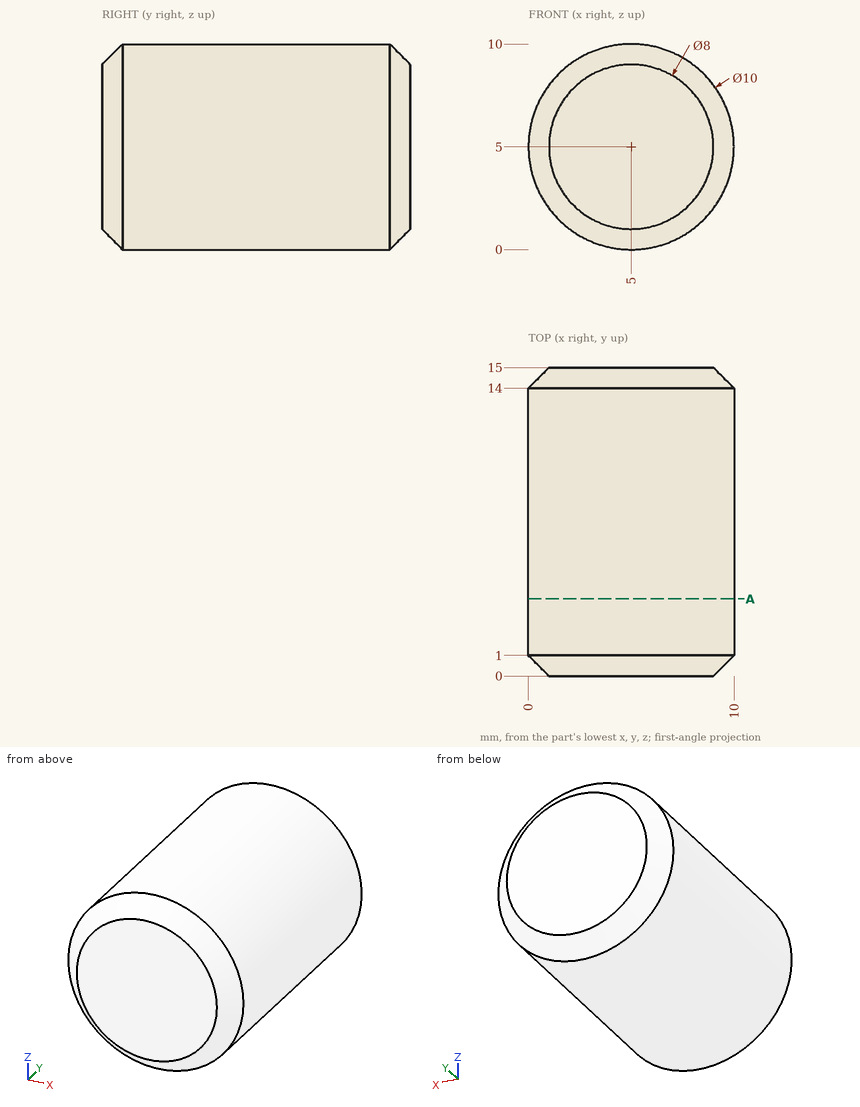
Could you check a few things on this drawing? It's one solid part, dimensions in mm from its lowest x, y, z. Give positions to 0.01 mm unless a question says otherwise; leave off trailing zeros. Loops run counter-clockwise (first coordinate to the right, second up) from the corner with the lowest first, then second, coordinate; pieces in that order, holes last. Notation, with made-up numbers: M -2,63.5 L 20,63.5 A24 cw 20,90.5 Z; hole C -28,67 d9. An arc over 180 degrees is marked long. Return JSON: item names as keys, results as strings.
Item 1: Imagine slicing it at A-A on y = 3.75. List the corners of the cut face in (x, z) for me.
A:
{"outline": "C 5,5 d10"}
Item 2: I'm going to push flat-ended pins straight in: pin 1 Ø4 at (y, z) = (9.5, 8.5) entering from +X; pin 2 Ø4 at (x, y) = (8.5, 5.5) entering from -Z. Where does each tip first touch, or does it pass through?
A:
{"pin 1": "stops at x = 9.77", "pin 2": "stops at z = 0.23"}
Item 3: Please list where these lines run through material, in increasing order: line 1 (X direction, y = 8.5, z = 2); line 2 (Z direction, x = 7.5, y = 0.5); line 3 (Z direction, x = 6, y = 4).
A:
{"line 1": "x = 1 to 9", "line 2": "z = 1.26 to 8.74", "line 3": "z = 0.1 to 9.9"}
